Geometry: final body of the model. Coordinates: model frame, mm. Coordinates: 2 decimals unless noted, no trailing zeros. Write each loop counter-clockwise with the first axis right and the second up, starting at its lowest first coordinate (ties: lowest second). Pieces come first, ordered by that corner, then holes. Notation, with made-up numbers: (33.5, -9.5) - (54.5, -9.5) arc R36 ccw to (54.5, 24.5) - close; hole circle Ø5 at (4.5, 67). An arc over 180 degrees is marked (long way). Answer as a JSON object with one key per item and string values. Group by question number.
Item 1: Line query: line 1 along X through (y, z) = (1.1, 5.75) (3 decimals); line 2 along Z through (x, y) = (-9, 0.3); line 3 along Z through (x, y) = (11, 1.25). Output: solid intervals per line, ascending. Write a range as from..to.
Item 2: Section B-B on z = -3. Return loops of the section in (x, y) (3 decimals), and give its area (3 significant figures).
Item 3: Section A-A on x = 4. Return loops of the section in (y, z), and give its area (3 significant figures).
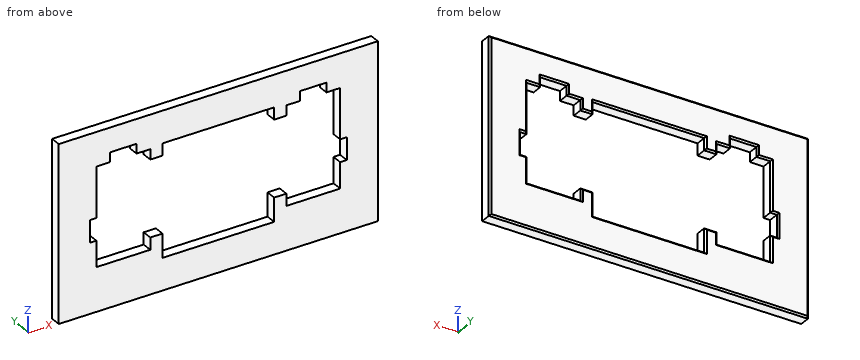
```python
from build123d import *

# Parameters (mm, degrees)
SKETCH1_W           = 40
SKETCH1_H           = 22
BOSS_EXTRUDE1_DEPTH = 1.5
CUT_EXTRUDE1_DEPTH  = 2.5
CHAMFER1_SIZE       = 0.2


with BuildPart() as part:
    # Sketch1 → Boss-Extrude1 (new body)
    with BuildSketch(Plane(origin=(0, 0, 0), x_dir=(1, 0, 0), z_dir=(0, 1, 0))):
        Rectangle(SKETCH1_W, SKETCH1_H)
    extrude(amount=BOSS_EXTRUDE1_DEPTH)

    # Sketch2 → Cut-Extrude1 (cut, through all)
    with BuildSketch(Plane(origin=(0, 1.5, 0), x_dir=(1, 0, 0), z_dir=(0, 1, 0))):
        Polygon((-7, 4.03), (-8.525, 4.03), (-8.525, 5.53), (-15.275, 5.53), (-15.275, 2.3), (-16.1, 2.3), (-16.1, -0.485), (-15.275, -0.485), (-15.275, -6.77), (-13.55, -6.77), (-13.55, -7.97), (-10.25, -7.97), (-10.25, -6.77), (-8.525, -6.77), (-8.525, -5.5), (-7, -5.5), (-7, -7), (7, -7), (7, -5.5), (8.525, -5.5), (8.525, -6.77), (10.25, -6.77), (10.25, -7.97), (13.55, -7.97), (13.55, -6.77), (15.275, -6.77), (15.275, -0.485), (16.1, -0.485), (16.1, 2.3), (15.275, 2.3), (15.275, 5.53), (8.525, 5.53), (8.525, 4.03), (7, 4.03), (7, 7), (-7, 7), align=None)
    extrude(amount=-CUT_EXTRUDE1_DEPTH, mode=Mode.SUBTRACT)

    # Chamfer1
    chamfer1_edges = [part.edges().sort_by_distance(p)[0] for p in [
        (-20, 1.5, 0),
        (0, 1.5, 11),
        (20, 1.5, 0),
        (7, 1.5, 6.25),
        (7.7625, 1.5, 5.5),
        (8.525, 1.5, 6.135),
        (9.3875, 1.5, 6.77),
        (10.25, 1.5, 7.37),
        (11.9, 1.5, 7.97),
        (13.55, 1.5, 7.37),
        (14.4125, 1.5, 6.77),
        (15.275, 1.5, 3.6275),
        (15.6875, 1.5, 0.485),
        (16.1, 1.5, -0.9075),
        (15.6875, 1.5, -2.3),
        (15.275, 1.5, -3.915),
        (11.9, 1.5, -5.53),
        (8.525, 1.5, -4.78),
        (7.7625, 1.5, -4.03),
        (7, 1.5, -5.515),
        (0, 1.5, -7),
        (-7, 1.5, -5.515),
        (-7.7625, 1.5, -4.03),
        (-8.525, 1.5, -4.78),
        (-11.9, 1.5, -5.53),
        (-15.275, 1.5, -3.915),
        (-15.6875, 1.5, -2.3),
        (-16.1, 1.5, -0.9075),
        (-15.6875, 1.5, 0.485),
        (-15.275, 1.5, 3.6275),
        (-14.4125, 1.5, 6.77),
        (-13.55, 1.5, 7.37),
        (-11.9, 1.5, 7.97),
        (-10.25, 1.5, 7.37),
        (-9.3875, 1.5, 6.77),
        (-8.525, 1.5, 6.135),
        (-7.7625, 1.5, 5.5),
        (-7, 1.5, 6.25),
        (0, 1.5, 7),
        (0, 1.5, -11),
    ]]
    chamfer(chamfer1_edges, length=CHAMFER1_SIZE)


solid = part.part
```
Checks:
{
 "1": {"line 1": "-20..-15.275, -8.525..-7, 7..8.525, 15.275..20", "line 2": "-11..-5.53, 6.77..11", "line 3": "-11..-5.53, 7.97..11"},
 "2": {"outline": "(-20, 0) - (-15.275, 0) - (-15.275, 1.3) - (-15.475, 1.5) - (-19.8, 1.5) - (-20, 1.3) - close; (15.275, 0) - (20, 0) - (20, 1.3) - (19.8, 1.5) - (15.475, 1.5) - (15.275, 1.3) - close", "area": "14.1 mm^2"},
 "3": {"outline": "(0, -11) - (1.3, -11) - (1.5, -10.8) - (1.5, -7.2) - (1.3, -7) - (0, -7) - close; (0, 7) - (1.3, 7) - (1.5, 7.2) - (1.5, 10.8) - (1.3, 11) - (0, 11) - close", "area": "11.9 mm^2"}
}
